from build123d import *

# Parameters (mm, degrees)
F0_W      = 45.2
F0_H      = 35.2
F1_DEPTH  = 18.35
F2_W      = 37.4
F2_H      = 35.2
F3_DEPTH  = 7.75
F4_W      = 45.2
F4_H      = 21
F5_DEPTH  = 6.5
F6_W      = 4.8
F6_H      = 6.25
F7_DEPTH  = 45.201
F8_W      = 3.5
F8_H      = 7
F9_DEPTH  = 45.201
F10_R     = 1.6
F11_DEPTH = 11.851


with BuildPart() as f1:
    # F0 (on Top) → F1 (new body)
    with BuildSketch(Plane.XY):
        Rectangle(F0_W, F0_H)
    extrude(amount=F1_DEPTH)

    # F2 (on face) → F3 (cut)
    with BuildSketch(Plane(origin=(0, 0, 0), x_dir=(1, 0, 0), z_dir=(0, 0, -1))):
        Rectangle(F2_W, F2_H)
    extrude(amount=-F3_DEPTH, mode=Mode.SUBTRACT)

    # F4 (on face) → F5 (cut)
    with BuildSketch(Plane.XY.offset(18.35)):
        Rectangle(F4_W, F4_H)
    extrude(amount=-F5_DEPTH, mode=Mode.SUBTRACT)

    # F6 (on face) → F7 (cut, through all)
    with BuildSketch(Plane(origin=(-22.6, 0, 0), x_dir=(0, -1, 0), z_dir=(-1, 0, 0))):
        with Locations((-15.2, 13.725)):
            Rectangle(F6_W, F6_H)
        with Locations((15.2, 13.725)):
            Rectangle(F6_W, F6_H)
    extrude(amount=-F7_DEPTH, mode=Mode.SUBTRACT)

    # F8 (on face) → F9 (cut, through all)
    with BuildSketch(Plane(origin=(-22.6, 0, 0), x_dir=(0, -1, 0), z_dir=(-1, 0, 0))):
        Polygon((-12.8, 16.85), (-17.6, 17.6), (-17.6, 16.85), align=None)
        Polygon((17.6, 16.85), (17.6, 17.6), (12.8, 16.85), align=None)
        with Locations((0, 5.5)):
            Rectangle(F8_W, F8_H)
    extrude(amount=-F9_DEPTH, mode=Mode.SUBTRACT)

    # F10 (on face) → F11 (cut, through all)
    with BuildSketch(Plane.XY.offset(11.85)):
        with Locations((15.5, -4.9)):
            Circle(F10_R)
        with Locations((-15.5, 4.9)):
            Circle(F10_R)
        with BuildLine():
            ThreePointArc((-16.5583005244, -4.9), (-16.9583005244, -5.4416994756), (-17.1, -6.1))
            ThreePointArc((-17.1, -6.1), (-15.5, -7.7), (-13.9, -6.1))
            ThreePointArc((-13.9, -6.1), (-14.0416994756, -5.4416994756), (-14.4416994756, -4.9))
            ThreePointArc((-14.4416994756, -4.9), (-15.5, -5.3), (-16.5583005244, -4.9))
        make_face()
        with BuildLine():
            Line((-17.1, -3.7), (-17.1, -6.1))
            ThreePointArc((-17.1, -6.1), (-16.9583005244, -5.4416994756), (-16.5583005244, -4.9))
            ThreePointArc((-16.5583005244, -4.9), (-16.9583005244, -4.3583005244), (-17.1, -3.7))
        make_face()
        with BuildLine():
            ThreePointArc((-14.4416994756, -4.9), (-14.0416994756, -5.4416994756), (-13.9, -6.1))
            Line((-13.9, -6.1), (-13.9, -3.7))
            ThreePointArc((-13.9, -3.7), (-14.0416994756, -4.3583005244), (-14.4416994756, -4.9))
        make_face()
        with BuildLine():
            ThreePointArc((-17.1, -3.7), (-16.9583005244, -4.3583005244), (-16.5583005244, -4.9))
            ThreePointArc((-16.5583005244, -4.9), (-15.5, -4.5), (-14.4416994756, -4.9))
            ThreePointArc((-14.4416994756, -4.9), (-14.0416994756, -4.3583005244), (-13.9, -3.7))
            ThreePointArc((-13.9, -3.7), (-15.5, -2.1), (-17.1, -3.7))
        make_face()
        with BuildLine():
            ThreePointArc((14.4416994756, 4.9), (14.0416994756, 4.3583005244), (13.9, 3.7))
            ThreePointArc((13.9, 3.7), (15.5, 2.1), (17.1, 3.7))
            ThreePointArc((17.1, 3.7), (16.9583005244, 4.3583005244), (16.5583005244, 4.9))
            ThreePointArc((16.5583005244, 4.9), (15.5, 4.5), (14.4416994756, 4.9))
        make_face()
        with BuildLine():
            Line((13.9, 6.1), (13.9, 3.7))
            ThreePointArc((13.9, 3.7), (14.0416994756, 4.3583005244), (14.4416994756, 4.9))
            ThreePointArc((14.4416994756, 4.9), (14.0416994756, 5.4416994756), (13.9, 6.1))
        make_face()
        with BuildLine():
            ThreePointArc((16.5583005244, 4.9), (16.9583005244, 4.3583005244), (17.1, 3.7))
            Line((17.1, 3.7), (17.1, 6.1))
            ThreePointArc((17.1, 6.1), (16.9583005244, 5.4416994756), (16.5583005244, 4.9))
        make_face()
        with BuildLine():
            ThreePointArc((13.9, 6.1), (14.0416994756, 5.4416994756), (14.4416994756, 4.9))
            ThreePointArc((14.4416994756, 4.9), (15.5, 5.3), (16.5583005244, 4.9))
            ThreePointArc((16.5583005244, 4.9), (16.9583005244, 5.4416994756), (17.1, 6.1))
            ThreePointArc((17.1, 6.1), (15.5, 7.7), (13.9, 6.1))
        make_face()
        with BuildLine():
            ThreePointArc((16.5583005244, 4.9), (15.5, 5.3), (14.4416994756, 4.9))
            ThreePointArc((14.4416994756, 4.9), (15.5, 4.5), (16.5583005244, 4.9))
        make_face()
        with BuildLine():
            ThreePointArc((-14.4416994756, -4.9), (-15.5, -4.5), (-16.5583005244, -4.9))
            ThreePointArc((-16.5583005244, -4.9), (-15.5, -5.3), (-14.4416994756, -4.9))
        make_face()
    extrude(amount=-F11_DEPTH, mode=Mode.SUBTRACT)


solid = f1.part
Can you work these out from the model? Positions are in its coordinate system, mm. A direction names the side the tool comes from. Give positions to 0.01 mm unless a question says otherwise; leave off trailing zeros. Order: outer loops, then holes, each group sorted by start corner. A loop starts at its lowest first (then second) coordinate and runs counter-clockwise, first axis right, second up. Notation, with made-up numbers: (-34.5, 48) - (-3.5, 48) arc R26 ccw to (-3.5, 69) - close; hole circle Ø9 at (30.5, -20). An arc over 180 degrees is marked (long way). Write each question's results on one line, items separated by ' | '.
1) I'm going to push flat-ended pins straight in: pin 1 Ø10 at (x, y) = (2.5, 10) entering from -Z; pin 2 Ø1 at (x, z) = (1.5, 12.5) entering from +Y; pin 3 Ø17 at (x, y) = (-9, 0.5) entering from +Z. Where does each tip first touch, or does it pass through?
Final values:
pin 1: stops at z = 7.75 | pin 2: stops at y = 12.8 | pin 3: stops at z = 11.85
2) If we mould it in two halves opening along Z, with no side actions, what happens to faces 4 (the face through (0, -1.75, 8)), 5 (the face through (0, 14, 18.35)), 6 (the face through (-18.7, 0, 1))? For each: pulls with the +Z half, pulls with the -Z half, needs draft (parallel to the pull), parting line crosses it, or undercut.
Final values:
face 4: undercut | face 5: pulls with the +Z half | face 6: needs draft
3) Suppose I cut it at A-A, the plane y = -4.9. Write out the boundary of the cut face in (x, z).
Final values:
outline: (-22.6, 0) - (-18.7, 0) - (-18.7, 7.75) - (-17.1, 7.75) - (-17.1, 11.85) - (-22.6, 11.85) - close; (-13.9, 7.75) - (13.9, 7.75) - (13.9, 11.85) - (-13.9, 11.85) - close; (17.1, 7.75) - (18.7, 7.75) - (18.7, 0) - (22.6, 0) - (22.6, 11.85) - (17.1, 11.85) - close
4) Suppose I cut it at D-D, the plane y = -11.5. Write out the boundary of the cut face in (x, z).
Final values:
outline: (-22.6, 0) - (-18.7, 0) - (-18.7, 7.75) - (18.7, 7.75) - (18.7, 0) - (22.6, 0) - (22.6, 18.35) - (-22.6, 18.35) - close
5) Suppose I cut it at C-C, the plane x = 15.5. Write out the boundary of the cut face in (y, z).
Final values:
outline: (-17.6, 7.75) - (-6.5, 7.75) - (-6.5, 11.85) - (-10.5, 11.85) - (-10.5, 18.35) - (-17.6, 18.35) - (-17.6, 17.6) - (-12.8, 16.85) - (-12.8, 10.6) - (-17.6, 10.6) - close; (-3.3, 7.75) - (-1.75, 7.75) - (-1.75, 9) - (1.75, 9) - (1.75, 7.75) - (2.1, 7.75) - (2.1, 11.85) - (-3.3, 11.85) - close; (7.7, 7.75) - (17.6, 7.75) - (17.6, 10.6) - (12.8, 10.6) - (12.8, 16.85) - (17.6, 17.6) - (17.6, 18.35) - (10.5, 18.35) - (10.5, 11.85) - (7.7, 11.85) - close
6) Suppose I cut it at B-B, the plane z = 13.5. Write out the boundary of the cut face in (x, y), then the cut area to 3 significant figures.
Final values:
outline: (-22.6, -12.8) - (22.6, -12.8) - (22.6, -10.5) - (-22.6, -10.5) - close; (-22.6, 10.5) - (22.6, 10.5) - (22.6, 12.8) - (-22.6, 12.8) - close | area: 208 mm^2
7) On a 3-axis mill with a long thin cutter (end or side, diameter ignored), from which of +Z, -Z, +X, -X, +Y, -Y can I reach the whole of each face in a straight line? I mean faces 1 (the face through (-15.5, -7.7, 9.8)), 2 (the face through (0, 10, 7.75)), 3 (the face through (21, 0, 2)). Say none if no direction works.
Final values:
face 1: +Z, -Z | face 2: -Z, +Y, -Y | face 3: +X, -X
8) Please list where these lines run through material, in increasing order: line 1 along Y through (x, z) = (15.5, 9.35); line 2 along Y through (x, z) = (-15.5, 8.7); line 3 along Y through (x, z) = (-5, 14). Write a range as [from, to].
Final values:
line 1: y = [-17.6, -6.5], [-3.3, 2.1], [7.7, 17.6] | line 2: y = [-17.6, -7.7], [-2.1, -1.75], [1.75, 3.3], [6.5, 17.6] | line 3: y = [-12.8, -10.5], [10.5, 12.8]
